Input: part model. Units: mm. Frame: model coordinates. A direction names the side the tool comes from. Give positions to 0.01 mm unless a question says otherwise; leave off trailing zeros. Loops run counter-clockwise (first coordinate to the right, second up) from the corner with the lowest first, then second, coordinate; pieces in that order, holes last. Notation, with made-up numbers: (-22, 16) - (27, 16) arc R12 cw to (27, 20) - close; hole circle Ø5 at (58.25, 24.25). An arc over 180 degrees is marked (long way). Answer as a JSON object with one key per item and string values.
from build123d import *

# Parameters (mm, degrees)
F0_W     = 177.00053
F0_H     = 75.980723
F1_DEPTH = 25
F2_W     = 141.91997
F2_H     = 34.842628
F3_DEPTH = 40
F4_R     = 5


with BuildPart() as f1:
    # F0 (on Top) → F1 (new body)
    with BuildSketch(Plane.XY):
        with Locations((1.726832, -3.02196)):
            Rectangle(F0_W, F0_H)
    extrude(amount=F1_DEPTH)

    # F2 (on face) → F3 (join)
    with BuildSketch(Plane.XY.offset(25)):
        with Locations((4.559569, -3.399281)):
            Rectangle(F2_W, F2_H)
    extrude(amount=F3_DEPTH)

    # F4
    f4_edges = [f1.edges().sort_by_distance(p)[0] for p in [
        (4.559569, -20.820595, 65),
        (-66.400416, -3.399281, 65),
        (4.559569, 14.022033, 65),
        (75.519554, -3.399281, 65),
    ]]
    fillet(f4_edges, radius=F4_R)


solid = f1.part
Item 1: Access query for faces 1 (the face through (4, -20.821, 42)), 2 (the face through (4, 14.022, 42)), 3 (the face through (75.52, -4, 42)). Directions: +Z, -Z, +X, -X, +Y, -Y. A direction counts if a zero-diameter tool reaches every point of the face in a straight line with its end or side. Return the directions, or none.
Geometry check:
{"face 1": "+Z, +X, -X, -Y", "face 2": "+Z, +X, -X, +Y", "face 3": "+Z, +X, +Y, -Y"}
Item 2: Cut plane C-C (z = 42). Return loops of the section in (x, y), then the cut area to 3 significant figures.
Geometry check:
{"outline": "(-66.4, -20.82) - (75.52, -20.82) - (75.52, 14.02) - (-66.4, 14.02) - close", "area": "4,940 mm2"}
Item 3: Contact query for flat-ended pins moving along their axis: P1, Ø6, axis at x = -55.5, z = 55.5, coming from the +Y side; P2, Ø3, axis at y = -10.5, z = 37, coming from the +X side; P3, Ø10.5, axis at x = 39.5, z = 49.5, coming from the -Y side. Output: stop coordinate, or through.
Geometry check:
{"P1": "stops at y = 14.02", "P2": "stops at x = 75.52", "P3": "stops at y = -20.82"}
Item 4: Cut plane D-D (x = -73). Return loops of the section in (y, z).
Geometry check:
{"outline": "(-41.01, 0) - (34.97, 0) - (34.97, 25) - (-41.01, 25) - close"}
Item 5: Material intervals for line 1 (Z direction, x = 43, y = 24); line 2 (Y direction, x = 5.5, z = 54); line 3 (X direction, y = -11, z = 35), sorted ascending. Write a range as [from, to].
Geometry check:
{"line 1": "z = [0, 25]", "line 2": "y = [-20.82, 14.02]", "line 3": "x = [-66.4, 75.52]"}
Item 6: Cut plane B-B (y = 6). Return loops of the section in (x, z), then the cut area to 3 significant figures.
Geometry check:
{"outline": "(-86.77, 0) - (90.23, 0) - (90.23, 25) - (75.52, 25) - (75.52, 60) arc R5 ccw to (70.52, 65) - (-61.4, 65) arc R5 ccw to (-66.4, 60) - (-66.4, 25) - (-86.77, 25) - close", "area": "10,100 mm2"}
Item 7: Cut plane A-A (x = -24). Return loops of the section in (y, z).
Geometry check:
{"outline": "(-41.01, 0) - (34.97, 0) - (34.97, 25) - (14.02, 25) - (14.02, 60) arc R5 ccw to (9.02, 65) - (-15.82, 65) arc R5 ccw to (-20.82, 60) - (-20.82, 25) - (-41.01, 25) - close"}
